Part model, mm, in its own coordinate system. Round coordinates to 2 decimals unless told otherwise and drop trailing zeros. Write each loop counter-clockwise with the first axis right and the second up, starting at its lowest first coordinate (ties: lowest second). Pieces come first, ordered by that corner, then holes. Notation, with made-up numbers: M 2.25,38.25 L 61.25,38.25 A26 cw 61.25,59.25 Z; hole C 35,77.5 d9. An arc over 180 degrees is marked long. Answer as a JSON object with one key per item and string values. Group by question number.
1. Drill centre lines: line 1 (Y direction, x = -2.25, z = 123); line 2 (Z direction, x = 2.5, y = 4); line 3 (Z direction, x = 0.25, y = 18.5). Where is each one in solid material? Low to high. Write a range as from..to.
2. Band-saw the part on A-A, the plane z = 187.5. Write the cut outline in (x, y), plus the area to 3 significant figures.
3. Drop flat-ended pins along their axis: pin 1 (3 mm diameter, centred on x = 1.5, y = 50, fed in from -Z); pin 2 (1.5 mm diameter, centred on x = 0.5, y = 23.5, fed in from +Z); pin 3 (4 mm diameter, centred on x = 3.5, y = 42, fed in from -Z). Give the stop position or say it passes through.
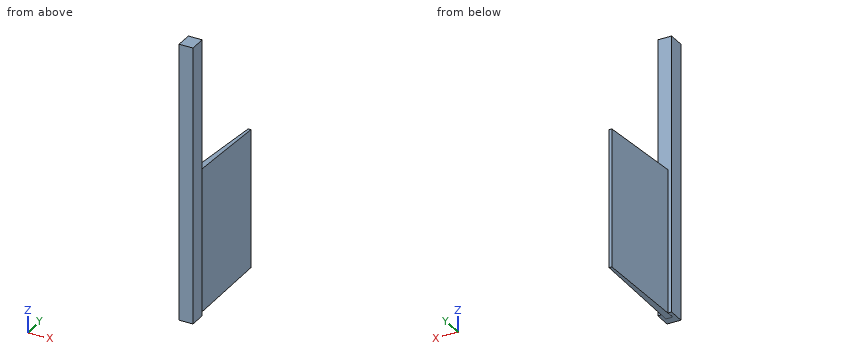
from build123d import *

# Parameters (mm, degrees)
ESQUISSE1_W        = 10
ESQUISSE1_H        = 12
BOSS_EXTRU_1_DEPTH = 200


with BuildPart() as part:
    # Esquisse1 → Boss.-Extru.1 (new body)
    with BuildSketch(Plane.XY):
        Rectangle(ESQUISSE1_W, ESQUISSE1_H)
    extrude(amount=BOSS_EXTRU_1_DEPTH)

    # Esquisse4 → Lissage2 section 0
    with BuildSketch(Plane(origin=(0, 0, 0), x_dir=(1, 0, 0), z_dir=(0, 1, 0))):
        with BuildLine():
            Line((-2.5, 0.020027966), (2.5, 0.020027966))
            Line((2.5, 0.020027966), (2.5, -104.18332506))
            Line((2.5, -104.18332506), (-2.5, -104.18332506))
            Line((-2.5, -104.18332506), (-2.5, 0.020027966))
        make_face()
    # Esquisse3 → Lissage2 section 1
    with BuildSketch(Plane(origin=(0, 76, 0), x_dir=(1, 0, 0), z_dir=(0, 1, 0))):
        with BuildLine():
            Line((-1, 0.876103951), (1, 0.876103951))
            Line((1, 0.876103951), (1, -99.123896049))
            Line((1, -99.123896049), (-1, -99.123896049))
            Line((-1, -99.123896049), (-1, 0.876103951))
        make_face()
    loft()


solid = part.part
Worked answers:
{
 "1": {"line 1": "y = -6..6", "line 2": "z = 0..200", "line 3": "z = -0.23..102.95"},
 "2": {"outline": "M -5,-6 L 5,-6 L 5,6 L -5,6 Z", "area": "120 mm^2"},
 "3": {"pin 1": "stops at z = -0.6", "pin 2": "stops at z = 102.67", "pin 3": "stops at z = -0.5"}
}
